Geometry: final body of the model. Coordinates: model frame, mm. Give positions to 0.01 mm unless a question says otherwise; leave off trailing zeros.
from build123d import *

# Parameters (mm, degrees)
F0_W      = 19.05
F0_H      = 1060.45
F1_DEPTH  = 609.6
F2_R      = 1.5875
F3_DEPTH  = 19.051
F4_R      = 1.5875
F5_DEPTH  = 25.4
F6_R      = 1.5875
F7_DEPTH  = 25.4
F8_R      = 1.5875
F9_DEPTH  = 25.4
F10_R     = 1.5875
F11_DEPTH = 19.051
F12_W     = 4.826
F12_H     = 15.875
F13_DEPTH = 1060.451
F14_W     = 4.826
F14_H     = 15.875
F15_DEPTH = 1060.451
F16_R     = 1.5875
F17_DEPTH = 1060.451


with BuildPart() as f1:
    # F0 (on Front) → F1 (new body)
    with BuildSketch(Plane.XZ):
        with Locations((9.525, 530.225)):
            Rectangle(F0_W, F0_H)
    extrude(amount=-F1_DEPTH)

    # F2 (on Right) → F3 (cut, through all)
    with BuildSketch(Plane.YZ):
        with Locations((50.8, 9.525)):
            Circle(F2_R)
        with Locations((177.8, 9.525)):
            Circle(F2_R)
        with Locations((304.8, 9.525)):
            Circle(F2_R)
        with Locations((431.8, 9.525)):
            Circle(F2_R)
        with Locations((558.8, 9.525)):
            Circle(F2_R)
    extrude(amount=F3_DEPTH, mode=Mode.SUBTRACT)

    # F4 (on Front) → F5 (cut)
    with BuildSketch(Plane.XZ):
        with Locations((9.525, 1054.1)):
            Circle(F4_R)
        with Locations((9.332581, 1028.700729)):
            Circle(F4_R)
    extrude(amount=-F5_DEPTH, mode=Mode.SUBTRACT)

    # F6 (on Front) → F7 (cut)
    with BuildSketch(Plane.XZ):
        with Locations((9.525, 6.35)):
            Circle(F6_R)
        with Locations((9.525, 31.75)):
            Circle(F6_R)
    extrude(amount=-F7_DEPTH, mode=Mode.SUBTRACT)

    # F8 (on Front) → F9 (cut)
    with BuildSketch(Plane.XZ):
        with Locations((9.525, 987.425)):
            Circle(F8_R)
        with Locations((9.525, 835.025)):
            Circle(F8_R)
        with Locations((9.525, 682.625)):
            Circle(F8_R)
        with Locations((9.525, 530.225)):
            Circle(F8_R)
        with Locations((9.525, 377.825)):
            Circle(F8_R)
        with Locations((9.525, 225.425)):
            Circle(F8_R)
        with Locations((9.525, 73.025)):
            Circle(F8_R)
    extrude(amount=-F9_DEPTH, mode=Mode.SUBTRACT)

    # F10 (on face) → F11 (cut, through all)
    with BuildSketch(Plane.YZ.offset(19.05)):
        with Locations((600.075, 1038.225)):
            Circle(F10_R)
        with Locations((600.075, 911.225)):
            Circle(F10_R)
        with Locations((600.075, 784.225)):
            Circle(F10_R)
        with Locations((600.075, 657.225)):
            Circle(F10_R)
        with Locations((600.075, 530.225)):
            Circle(F10_R)
        with Locations((600.075, 403.225)):
            Circle(F10_R)
        with Locations((600.075, 276.225)):
            Circle(F10_R)
        with Locations((600.075, 149.225)):
            Circle(F10_R)
        with Locations((600.075, 22.225)):
            Circle(F10_R)
    extrude(amount=-F11_DEPTH, mode=Mode.SUBTRACT)

    # F12 (on face) → F13 (cut, through all)
    with BuildSketch(Plane(origin=(0, 0, 0), x_dir=(1, 0, 0), z_dir=(0, 0, -1))):
        with Locations((16.637, -109.5375)):
            Rectangle(F12_W, F12_H)
    extrude(amount=-F13_DEPTH, mode=Mode.SUBTRACT)

    # F14 (on face) → F15 (cut, through all)
    with BuildSketch(Plane(origin=(0, 0, 0), x_dir=(1, 0, 0), z_dir=(0, 0, -1))):
        with Locations((16.637, -500.0625)):
            Rectangle(F14_W, F14_H)
    extrude(amount=-F15_DEPTH, mode=Mode.SUBTRACT)

    # F16 (on Top) → F17 (cut, through all)
    with BuildSketch(Plane.XY):
        with Locations((9.525, 50.8)):
            Circle(F16_R)
        with Locations((9.525, 304.8)):
            Circle(F16_R)
        with Locations((9.525, 558.8)):
            Circle(F16_R)
    extrude(amount=F17_DEPTH, mode=Mode.SUBTRACT)


solid = f1.part
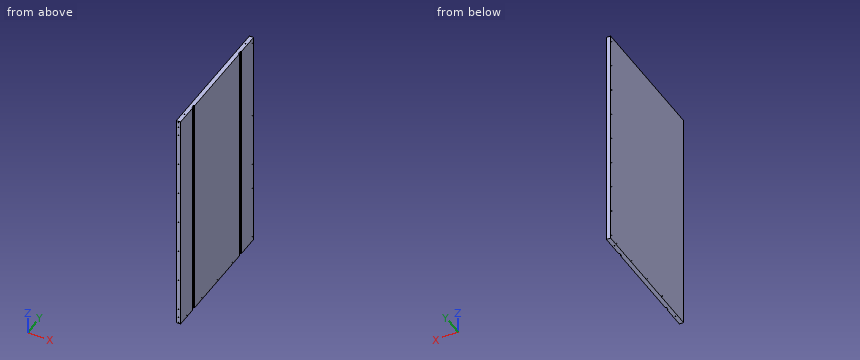
Item 1: Pin query (flat end, axial travel): pin 1 (8 mm diameter, centred on y = 501.5, z = 451, fed in from +X); pin 2 (1.6 mm diameter, centred on x = 10, z = 530, fed in from -Y); pin 3 (2.5 mm diameter, centred on y = 50.8, z = 9.525, fed in from -X). Return the tip coordinate at first contact, or that it passes through.
Values follow:
pin 1: stops at x = 14.22
pin 2: stops at y = 25.4
pin 3: passes through
Item 2: Section query A-A on z = 940. Give the number of separate pieces and of enclosed holes in the cut face, plus the area to 3 significant figures.
Values follow:
separate pieces: 1
enclosed holes: 3
area: 11,400 mm2
Item 3: Ray query, probe 1 along X at (y, z) = (50, 3); probe 2 along Y at (x, z) = (16.5, 197) (3 decimals); probe 3 along Z at (x, y) = (2.5, 558.8). Return the intervals inside material, ascending.
Values follow:
probe 1: x = 0 to 8.15, 10.9 to 19.05
probe 2: y = 0 to 101.6, 117.475 to 492.125, 508 to 609.6
probe 3: z = 0 to 7.94, 11.11 to 1060.45
